Design review of the part built by this model. Coordinates are the model's own, in mm. A direction names the side the tool comes from. Round coordinates to 2 decimals unless told otherwise and drop trailing zeros. Loops run counter-clockwise (first coordinate to the right, second up) from the corner with the lowest first, then second, coordinate; pieces in that order, holes last. Notation, with made-up numbers: (-15.75, 22) - (22.25, 22) arc R16 ccw to (22.25, 49) - close; hole circle Ø3 at (79.5, 25). An arc over 180 degrees is marked (long way). Return JSON: item names as keys, results as strings. Group by question number.
from build123d import *

# Parameters (mm, degrees)
SKETCH1_W            = 1680
SKETCH1_H            = 351
BASE_FLANGE1_DEPTH   = 1.5
EDGE_FLANGE1_START   = -644.471153846
EDGE_FLANGE1_DEPTH   = 1680
EDGE_FLANGE1_2_DEPTH = 1680
SKETCH9_R            = 2.5
CUT_EXTRUDE1_DEPTH   = 10


# Read off the part's stored shape, not the designer's step: Edge-Flange1
# Sheet-metal steps are written as plain solids
with BuildPart() as part:
    # Sketch1 → Base-Flange1 (new body)
    with BuildSketch(Plane.XY):
        with Locations((195.528846154, -50.139423077)):
            Rectangle(SKETCH1_W, SKETCH1_H)
    extrude(amount=-BASE_FLANGE1_DEPTH)

    # Edge-Flange1 outline → Edge-Flange1 (cut)
    with BuildSketch(Plane.YZ.offset(EDGE_FLANGE1_START)):
        with BuildLine():
            ThreePointArc((-215.175321462, -1.5), (-216.795506637, -1.102418412), (-218.047602785, 0))
            Line((-218.047602785, 0), (-225.639423077, 0))
            Line((-225.639423077, 0), (-225.639423077, -1.5))
            Line((-225.639423077, -1.5), (-215.175321462, -1.5))
        make_face()
    extrude(amount=EDGE_FLANGE1_DEPTH, mode=Mode.SUBTRACT)

    # Edge-Flange1 2 outline → Edge-Flange1 2 (add)
    with BuildSketch(Plane.YZ.offset(EDGE_FLANGE1_START)):
        with BuildLine():
            Line((-215.247118232, 6), (-216.925321462, 5.031088913))
            ThreePointArc((-216.925321462, 5.031088913), (-218.591362309, 2.762013733), (-218.047602785, 0))
            Line((-218.047602785, 0), (-215.175321462, 0))
            ThreePointArc((-215.175321462, 0), (-217.107173114, 1.48236191), (-216.175321462, 3.732050808))
            Line((-216.175321462, 3.732050808), (-214.497118232, 4.700961894))
            Line((-214.497118232, 4.700961894), (-215.247118232, 6))
        make_face()
    extrude(amount=EDGE_FLANGE1_2_DEPTH)

    # Sketch9 → Cut-Extrude1 (cut)
    with BuildSketch(Plane.XY):
        with Locations((-144.471153846, -14.639423077)):
            Circle(SKETCH9_R)
        with Locations((-144.471153846, -84.639423077)):
            Circle(SKETCH9_R)
        with Locations((535.528846154, -84.639423077)):
            Circle(SKETCH9_R)
        with Locations((535.528846154, -14.639423077)):
            Circle(SKETCH9_R)
        with BuildLine():
            Line((869.528846154, 125.360576923), (869.528846154, 109.360576923))
            ThreePointArc((869.528846154, 109.360576923), (865.528846154, 105.360576923), (861.528846154, 109.360576923))
            Line((861.528846154, 109.360576923), (861.528846154, 125.360576923))
            ThreePointArc((861.528846154, 125.360576923), (865.528846154, 129.360576923), (869.528846154, 125.360576923))
        make_face()
        with BuildLine():
            Line((199.528846154, 125.360576923), (199.528846154, 109.360576923))
            ThreePointArc((199.528846154, 109.360576923), (195.528846154, 105.360576923), (191.528846154, 109.360576923))
            Line((191.528846154, 109.360576923), (191.528846154, 125.360576923))
            ThreePointArc((191.528846154, 125.360576923), (195.528846154, 129.360576923), (199.528846154, 125.360576923))
        make_face()
        with BuildLine():
            Line((-470.471153846, 125.360576923), (-470.471153846, 109.360576923))
            ThreePointArc((-470.471153846, 109.360576923), (-474.471153846, 105.360576923), (-478.471153846, 109.360576923))
            Line((-478.471153846, 109.360576923), (-478.471153846, 125.360576923))
            ThreePointArc((-478.471153846, 125.360576923), (-474.471153846, 129.360576923), (-470.471153846, 125.360576923))
        make_face()
    extrude(amount=-CUT_EXTRUDE1_DEPTH, mode=Mode.SUBTRACT)


solid = part.part
Q1. Add section C-C, the plane y = 43.5. State the section outline as (x, z) points.
Q2. Insertion check: pin 1 Ø4 at (x, y) = (506, -162.5) entering from +Z; pin 2 Ø1 at (x, z) = (-364.5, 0.5) entering from -Y. Each pin has a flat end and moves straight along its axis. Give the tip position at first contact, or say it passes through.
Q3. For line 1 (Y direction, x = 147.5, z = 3.25); line 2 (Y direction, x = 172, z = 2.25); line 3 (Z direction, x = -59.5, y = 56.5), list the stretches that pass through material, from the lowest coordinate up.
Q4. Add section B-B, the plane z = 2. State the section outline as (x, y) points.
Q5. Tool access review of faces 1 (the flat face through (184, -43, 0)), 2 (the flat face through (184, -43, -1.5)): name each direction out of +Z, -Z, +X, -X, +Y, -Y from which nothing blocks a thin tool from reaching the whole face with its end or side.
Q6. Add section A-A, the plane x = 817.5. State the section outline as (y, z) points.
Evaluation:
{
 "1": {"outline": "(-644.47, -1.5) - (1035.53, -1.5) - (1035.53, 0) - (-644.47, 0) - close"},
 "2": {"pin 1": "z = 0", "pin 2": "y = -218.53"},
 "3": {"line 1": "-218.44 to -216.74", "line 2": "-218.67 to -217.16", "line 3": "-1.5 to 0"},
 "4": {"outline": "(-644.47, -218.68) - (1035.53, -218.68) - (1035.53, -217.18) - (-644.47, -217.18) - close"},
 "5": {"face 1": "+Z, +X, -X, +Y", "face 2": "-Z, +X, -X, +Y, -Y"},
 "6": {"outline": "(-216.93, 5.03) arc R3.5 ccw to (-215.18, -1.5) - (125.36, -1.5) - (125.36, 0) - (-215.18, 0) arc R2 cw to (-216.18, 3.73) - (-214.5, 4.7) - (-215.25, 6) - close"}
}
